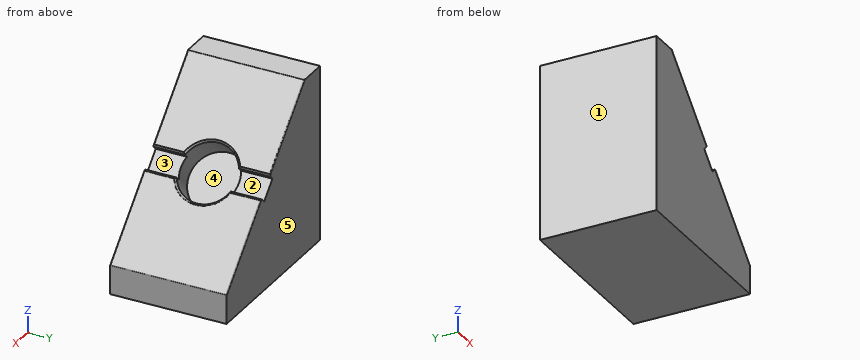
```python
from build123d import *

# Parameters (mm, degrees)
F1_DEPTH      = 50.8
F1_DEPTH_BACK = 50.8
F2_R          = 25.4
F3_DEPTH      = 25.4
F4_W          = 110.558038988
F4_H          = 19.05
F5_DEPTH      = 6.35
F6_SIZE       = 1.524
F7_R          = 0.762


with BuildPart() as f1:
    # F0 (on Front) → F1 (new body, two sides)
    with BuildSketch(Plane.XZ) as f1_sk:
        Polygon((0, 152.4), (0, 0), (152.4, 0), (152.4, 25.4), (25.4, 152.4), align=None)
    extrude(amount=F1_DEPTH)
    extrude(f1_sk.sketch, amount=-F1_DEPTH_BACK)

    # F2 (on face) → F3 (cut)
    with BuildSketch(Plane(origin=(88.9, 0, 88.9), x_dir=(0, 1, 0), z_dir=(0.7071067812, 0, 0.7071067812))):
        Circle(F2_R)
    extrude(amount=-F3_DEPTH, mode=Mode.SUBTRACT)

    # F4 (on face) → F5 (cut)
    with BuildSketch(Plane(origin=(88.9, 0, 88.9), x_dir=(0, 1, 0), z_dir=(0.7071067812, 0, 0.7071067812))):
        Rectangle(F4_W, F4_H)
    extrude(amount=-F5_DEPTH, mode=Mode.SUBTRACT)

    # F6
    f6_edges = [f1.edges().sort_by_distance(p)[0] for p in [
        (82.164808, -37.173215, 95.635192),
        (95.635192, -37.173215, 82.164808),
        (95.635192, 37.173215, 82.164808),
        (82.164808, 37.173215, 95.635192),
        (70.939488, 0, 106.860512),
        (106.860512, 0, 70.939488),
    ]]
    chamfer(f6_edges, length=F6_SIZE)

    # F7
    f7_edges = [f1.edges().sort_by_distance(p)[0] for p in [
        (25.4, 0, 152.4),
        (53.243589, -50.8, 124.556411),
        (53.243589, 50.8, 124.556411),
        (124.556411, 50.8, 53.243589),
        (96.712823, 37.67621, 81.087177),
        (152.4, 0, 25.4),
        (107.938143, 0, 69.861857),
        (124.556411, -50.8, 53.243589),
        (96.712823, -37.67621, 81.087177),
    ]]
    fillet(f7_edges, radius=F7_R)


solid = f1.part
```
CAD build for the part. Positions are in the model's coordinates, mm. Face numbers are marked on the shaded views. A direction names the side the tool comes from. Give positions to 0.01 mm unless a question says otherwise; leave off trailing zeros. Loops run counter-clockwise (first coordinate to the right, second up) from the corner with the lowest first, then second, coordinate; pieces in that order, holes last. Notation, with made-up numbers: (68, 49) - (96, 49) arc R13 cw to (96, 57) - close; hole circle Ø7 at (10.25, 45.25). An arc over 180 degrees is marked (long way). Put each result on its own line as item: value.
Q1. Flat gauge pins, fed straight in: pin 1 (1.1 mm diameter, centred on y = -31.5, z = 95.5, fed in from +X); pin 2 (1.5 mm diameter, centred on x = 95.5, y = 38.5, fed in from +Z); pin 3 (2 mm diameter, centred on x = 105, y = -1, fed in from -Z); pin 4 (3 mm diameter, centred on y = 19, z = 39.5, fed in from +X). Where does each tip first touch, or does it go through?
Filled in:
pin 1: stops at x = 81.09
pin 2: stops at z = 81.09
pin 3: stops at z = 0
pin 4: stops at x = 139.8
Q2. Tool access for the marked faces 1 and 2: list every direction of +Z, -Z, +X, -X, +Y, -Y with a clear straight run to the whole face (end or side of a thin tool).
Filled in:
face 1: +Z, -Z, -X, +Y, -Y
face 2: +Y, -Y
Q3. Mould opens along Y. For the marked faces 3, 4 and 5 say: pulls with the +Y half, pulls with the -Y half, needs draft (parallel to the pull), parting line crosses it, or undercut.
Filled in:
face 3: needs draft
face 4: undercut
face 5: pulls with the +Y half
Q4. Slice it at A-A (y = 43.5). Give the cut face in (x, z), plus the area to 3 significant figures.
Filled in:
outline: (0, 0) - (152.4, 0) - (152.4, 25.08) arc R0.76 ccw to (152.18, 25.62) - (96.94, 80.86) arc R0.76 ccw to (96.4, 81.09) - (94.56, 81.09) - (91.15, 77.67) - (77.67, 91.15) - (81.09, 94.56) - (81.09, 96.71) - (25.62, 152.18) arc R0.76 ccw to (25.08, 152.4) - (0, 152.4) - close
area: 15,000 mm²
Q5. Probe line 1 along Y through (x, z) = (143, 34); line 2 along X through (y, z) = (-20, 62); line 3 along Z through (x, y) = (88, 41). List the from-to ranges inside material, lowest first.
Filled in:
line 1: y = -50.77 to 50.77
line 2: x = 0 to 79.88, 84.14 to 115.8
line 3: z = 0 to 80.82
